Geometry check sheet. Reference: the model listing, model coordinates, mm. Give positions to 0.01 mm unless a question says otherwise; leave off trailing zeros. Loops run counter-clockwise (first coordinate to the right, second up) from the corner with the lowest first, then second, coordinate; pieces in that order, holes last. Notation, with made-up numbers: (26.5, 9) -> (43.5, 9) arc R21 ccw to (43.5, 47) -> close; hole circle Ø9 at (-40, 27.5). An arc over 180 degrees is marked (long way). Write item = value, one per line.
```python
from build123d import *

# Parameters (mm, degrees)
RESSALTO_EXTRUS_O1_DEPTH = 4
FURO_COM_FOLGA_DE_M31_D  = 3.2
FILETE1_R                = 3
M3_CLEARANCE_HOLE1_D     = 3.2
FURO_COM_FOLGA_DE_M32_D  = 2.87
M3_CLEARANCE_HOLE2_D     = 3.2
SKETCH3_W                = 27.430623534
SKETCH3_H                = 190
CUT_EXTRUDE1_DEPTH       = 10
BOSS_EXTRUDE1_DEPTH      = 4
FILLET3_R                = 3
BOSS_EXTRUDE3_DEPTH      = 4
M3_CLEARANCE_HOLE4_D     = 3.2
FILLET5_R                = 3
M5_CLEARANCE_HOLE1_D     = 5.3
SKETCH15_R               = 3
CUT_EXTRUDE6_DEPTH       = 5
SKETCH17_W               = 196
SKETCH17_H               = 23.942856981
CUT_EXTRUDE8_DEPTH       = 5
M3_CLEARANCE_HOLE5_D     = 3.2


with BuildPart() as part:
    # Esboço1 → Ressalto-extrusão1 (new body)
    with BuildSketch(Plane.XY):
        with BuildLine():
            Line((168.243612151, -138.115636704), (-79.756387849, -138.115636704))
            ThreePointArc((-79.756387849, -138.115636704), (-80.46349463, -137.822743485), (-80.756387849, -137.115636704))
            Line((-80.756387849, -137.115636704), (-80.756387849, 48.884363296))
            ThreePointArc((-80.756387849, 48.884363296), (-79.877708192, 51.005683639), (-77.756387849, 51.884363296))
            Line((-77.756387849, 51.884363296), (166.243612151, 51.884363296))
            ThreePointArc((166.243612151, 51.884363296), (168.364932495, 51.005683639), (169.243612151, 48.884363296))
            Line((169.243612151, 48.884363296), (169.243612151, -137.115636704))
            ThreePointArc((169.243612151, -137.115636704), (168.950718933, -137.822743485), (168.243612151, -138.115636704))
        make_face()
        with BuildLine():
            Line((-36.756387849, -93.115636704), (-55.756387849, -93.115636704))
            Line((-55.756387849, -93.115636704), (-55.756387849, -79.115636704))
            Line((-55.756387849, -79.115636704), (-55.756387849, 27.884363296))
            ThreePointArc((-55.756387849, 27.884363296), (-54.877708192, 30.005683639), (-52.756387849, 30.884363296))
            Line((-52.756387849, 30.884363296), (141.243612151, 30.884363296))
            ThreePointArc((141.243612151, 30.884363296), (143.364932495, 30.005683639), (144.243612151, 27.884363296))
            Line((144.243612151, 27.884363296), (144.243612151, -79.115636704))
            Line((144.243612151, -79.115636704), (144.243612151, -93.115636704))
            Line((144.243612151, -93.115636704), (125.243612151, -93.115636704))
            Line((125.243612151, -93.115636704), (125.243612151, -107.115636704))
            ThreePointArc((125.243612151, -107.115636704), (124.950718933, -107.822743485), (124.243612151, -108.115636704))
            Line((124.243612151, -108.115636704), (-35.756387849, -108.115636704))
            ThreePointArc((-35.756387849, -108.115636704), (-36.46349463, -107.822743485), (-36.756387849, -107.115636704))
            Line((-36.756387849, -107.115636704), (-36.756387849, -93.115636704))
        make_face(mode=Mode.SUBTRACT)
    extrude(amount=RESSALTO_EXTRUS_O1_DEPTH)

    # Furo com folga de M31 (through all)
    with Locations(Plane(origin=(0, 0, 0), x_dir=(-1, 0, 0), z_dir=(0, 0, -1))):
        with Locations((-148.743612151, -78.347886704), (-148.743612151, -18.347886704), (-148.743612151, 41.652113296), (60.256387849, 41.652113296), (60.256387849, -18.347886704), (60.256387849, -78.347886704), (72.956387849, 27.018533744), (72.956387849, -65.481466256), (19.656387849, -65.481466256), (19.656387849, 27.018533744)):
            Hole(FURO_COM_FOLGA_DE_M31_D / 2)

    # Filete1
    filete1_edges = [part.edges().sort_by_distance(p)[0] for p in [
        (-55.756387849, -93.115636704, 2),
        (-36.756387849, -93.115636704, 2),
        (125.243612151, -93.115636704, 2),
        (144.243612151, -93.115636704, 2),
    ]]
    fillet(filete1_edges, radius=FILETE1_R)

    # M3 Clearance Hole1 (through all)
    with Locations(Plane(origin=(0, 0, 0), x_dir=(-1, 0, 0), z_dir=(0, 0, -1))):
        with Locations((-164.230041881, -97.102981335), (43.669958119, -97.102981335), (75.742817578, -97.102981335)):
            Hole(M3_CLEARANCE_HOLE1_D / 2)

    # Furo com folga de M32 (through all)
    with Locations(Plane.XY.offset(4)):
        with Locations((44.243612151, 46.98714614)):
            Hole(FURO_COM_FOLGA_DE_M32_D / 2)

    # M3 Clearance Hole2 (through all)
    with Locations(Plane.XY.offset(4)):
        with Locations((161.560317261, 35.480164232), (161.560317261, 4.480164232)):
            Hole(M3_CLEARANCE_HOLE2_D / 2)

    # Sketch3 → Cut-Extrude1 (cut)
    with BuildSketch(Plane.XY.offset(4)):
        with Locations((169.958923918, -43.115636704)):
            Rectangle(SKETCH3_W, SKETCH3_H)
    extrude(amount=-CUT_EXTRUDE1_DEPTH, mode=Mode.SUBTRACT)

    # Sketch5 → Boss-Extrude1 (add)
    with BuildSketch(Plane(origin=(0, 0, 0), x_dir=(-1, 0, 0), z_dir=(0, 0, -1))):
        with BuildLine():
            Line((-145.240285588, -97.500155699), (-140.243612151, -97.500155699))
            Line((-140.243612151, -97.500155699), (-140.243612151, 27.941506315))
            ThreePointArc((-140.243612151, 27.941506315), (-139.345176367, 30.025791601), (-137.244155982, 30.884363296))
            Line((-137.244155982, 30.884363296), (-145.240285588, 30.884363296))
            Line((-145.240285588, 30.884363296), (-145.240285588, -97.500155699))
        make_face()
    extrude(amount=-BOSS_EXTRUDE1_DEPTH)

    # Fillet3
    fillet3_edges = [part.edges().sort_by_distance(p)[0] for p in [
        (156.243612151, 51.884363296, 2),
    ]]
    fillet(fillet3_edges, radius=FILLET3_R)

    # Sketch10 → Boss-Extrude3 (add)
    with BuildSketch(Plane(origin=(0, 0, 0), x_dir=(-1, 0, 0), z_dir=(0, 0, -1))):
        with BuildLine():
            Line((-156.243612151, -138.115636704), (-156.243612151, 48.884363296))
            ThreePointArc((-156.243612151, 48.884363296), (-155.364932495, 51.005683639), (-153.243612151, 51.884363296))
            Line((-153.243612151, 51.884363296), (-163.743612151, 51.884363296))
            Line((-163.743612151, 51.884363296), (-163.743612151, -138.115636704))
            Line((-163.743612151, -138.115636704), (-156.243612151, -138.115636704))
        make_face()
    extrude(amount=-BOSS_EXTRUDE3_DEPTH)

    # M3 Clearance Hole4 (through all)
    with Locations(Plane(origin=(0, 0, 0), x_dir=(-1, 0, 0), z_dir=(0, 0, -1))):
        with Locations((-160.743612151, -101.615636704), (-160.743612151, -132.615636704), (-129.743612151, -132.615636704), (-129.743612151, -101.615636704)):
            Hole(M3_CLEARANCE_HOLE4_D / 2)

    # Fillet5
    fillet5_edges = [part.edges().sort_by_distance(p)[0] for p in [
        (140.243612151, -93.115636704, 2),
        (163.743612151, 51.884363296, 2),
    ]]
    fillet(fillet5_edges, radius=FILLET5_R)

    # M5 Clearance Hole1 (through all)
    with Locations(Plane(origin=(0, 0, 0), x_dir=(-1, 0, 0), z_dir=(0, 0, -1))):
        with Locations((-115.03361215, -125.8856367), (26.54638785, -125.8856367), (-44.189907873, -129.865636704)):
            Hole(M5_CLEARANCE_HOLE1_D / 2)

    # Sketch15 → Cut-Extrude6 (cut, through all)
    with BuildSketch(Plane(origin=(0, 0, 0), x_dir=(-1, 0, 0), z_dir=(0, 0, -1))):
        with Locations((-145.243612151, -117.115636704)):
            Circle(SKETCH15_R)
    extrude(amount=-CUT_EXTRUDE6_DEPTH, mode=Mode.SUBTRACT)

    # Sketch17 → Cut-Extrude8 (cut)
    with BuildSketch(Plane(origin=(0, 0, 0), x_dir=(-1, 0, 0), z_dir=(0, 0, -1))):
        with Locations((-42.243612151, 39.912934806)):
            Rectangle(SKETCH17_W, SKETCH17_H)
    extrude(amount=-CUT_EXTRUDE8_DEPTH, mode=Mode.SUBTRACT)

    # M3 Clearance Hole5 (through all)
    with Locations(Plane.XY.offset(4)):
        with Locations((-75.756387849, 41.652113296), (-75.756387849, 48.152113296), (158.743612151, 48.152113296), (158.743612151, 41.652113296)):
            Hole(M3_CLEARANCE_HOLE5_D / 2)


solid = part.part
```
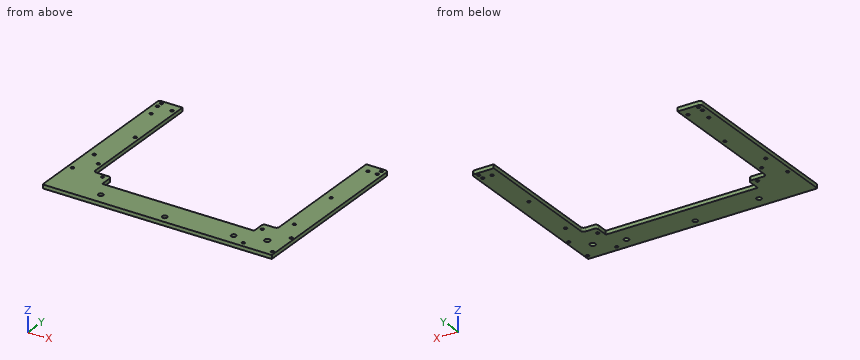
Item 1: Thickness scan on L1, parallel to X at y = -14, z = 1; L2, parallel to X at y = -117, z = 3; L3, parallel to X at y = -124, z = 2.8. Record the ranges inside material, lowest first. Write a range as [from, to].
Answer:
L1 = [-80.76, -55.76], [140.24, 163.74]
L2 = [-80.76, 142.25], [148.24, 163.74]
L3 = [-80.76, -28.41], [-24.68, 113.17], [116.9, 163.74]
Item 2: Section check A-A, the plane y = -27. Record the cut outline in (x, z), plus the area to 3 significant figures.
Answer:
outline = (-80.76, 0) -> (-55.76, 0) -> (-55.76, 4) -> (-80.76, 4) -> close; (140.24, 0) -> (163.74, 0) -> (163.74, 4) -> (140.24, 4) -> close
area = 194 mm^2
Item 3: Section check B-B, the plane x = 58. Record the cut outline in (y, z).
Answer:
outline = (-138.12, 0) -> (-108.12, 0) -> (-108.12, 4) -> (-138.12, 4) -> close
Item 4: Gauge pin test, flat end, axial feed: pin 1 (1.9 mm diameter, centred on x = -75.76, y = 41.65, fed in from +Z). Record the tip position at first contact, or that the pin passes through.
Answer:
pin_1 = through
Item 5: Section check C-C, the plane z = 3.3. Give the number of separate pieces and of enclosed holes in the cut face, plus the area to 3 significant figures.
Answer:
separate_pieces = 1
enclosed_holes = 22
area = 15,400 mm^2
